Check sheet for the drawn part. Datum: minimum x, y, z corner. Units: mm. A direction names the side the tool comes from. Coordinates: 2 decimals unless noted, no trailing zeros. Loops run counter-clockwise (first coordinate to the right, second up) from the corner with the lowest first, then second, coordinate; pieces in that order, holes last.
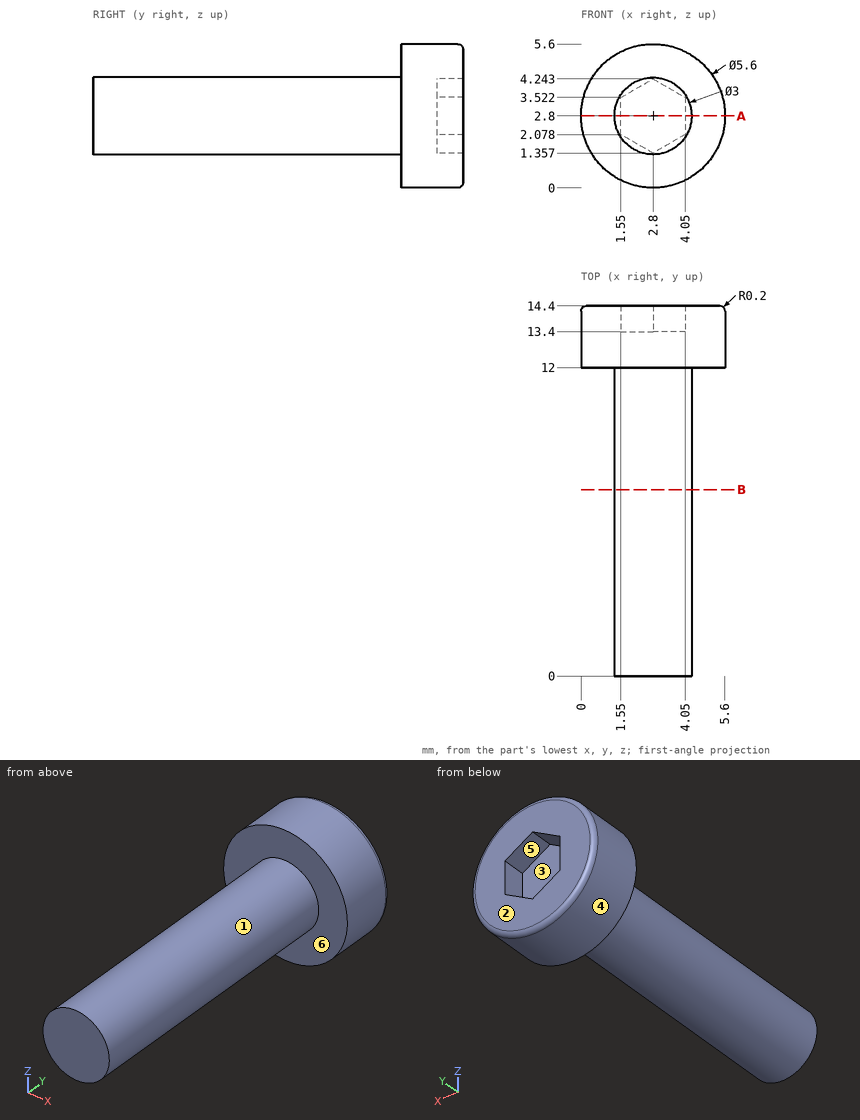
(1) Sectioned sample at B-B on y = 7.25. Record the cut outline in (x, z).
Findings:
outline: circle Ø3 at (2.8, 2.8)
(2) Draft check along Z on the marked faces 1, 2 and 3. Enter one of: +Z half, -Z half, draft (parallel to the pull), parting line (faces both ways), or undercut.
Findings:
face 1: parting line
face 2: draft
face 3: undercut
(3) Sectioned sample at A-A on z = 2.8. Record the cut outline in (x, y).
Findings:
outline: (0, 12) - (1.3, 12) - (1.3, 0) - (4.3, 0) - (4.3, 12) - (5.6, 12) - (5.6, 14.2) arc R0.2 ccw to (5.4, 14.4) - (4.05, 14.4) - (4.05, 13.4) - (1.55, 13.4) - (1.55, 14.4) - (0.2, 14.4) arc R0.2 ccw to (0, 14.2) - close
(4) Gauge pin test, flat ends, axial feed: pin 1 Ø2 at (x, z) = (1, 4) entering from -Y; pin 2 Ø2 at (x, y) = (4.5, 9.5) entering from -Z; pin 3 Ø1.5 at (y, z) = (1.5, 1) entering from -X; pin 4 Ø1.3 at (x, z) = (3, 2.5) entering from +Y. Record the tip position at first contact, or that the pin passes through.
Findings:
pin 1: stops at y = 0
pin 2: stops at z = 1.47
pin 3: stops at x = 1.73
pin 4: stops at y = 13.4
(5) Access from +Z, -Z, +X, -X, +Y, -Y to the whole of each face (thin tool, end or side, straight path). Record for the marked faces 4, 5 and 6.
Findings:
face 4: +Y, -Y
face 5: +Y
face 6: -Y
(6) Scan lines: L1, parallel to Y at x = 3.95, z = 0.7; L2, parallel to Y at x = 2.75, z = 2.55; L3, parallel to X at y = 4.25, z = 2.85. Record each from-to range of solid material in increasing order.
Findings:
L1: y = 12 to 14.4
L2: y = 0 to 13.4
L3: x = 1.3 to 4.3
